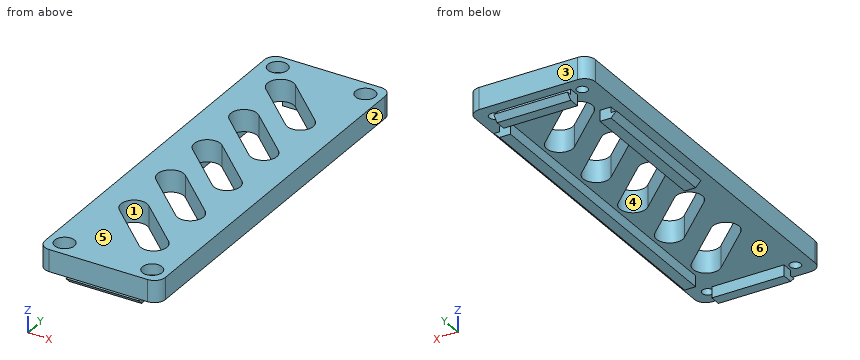
```python
from build123d import *

# Parameters (mm, degrees)
SKETCH_1_W          = 11
SKETCH_1_H          = 35
EXTRUDE_1_DEPTH     = 2
FILLET_1_R          = 1
SKETCH_2_W          = 1
SKETCH_2_H          = 27.801195883
SKETCH_2_H_2        = 12.696804569
SKETCH_2_W_2        = 6.728012357
SKETCH_2_H_3        = 1
SKETCH_2_W_3        = 6.596948746
EXTRUDE_2_DEPTH     = 1
SKETCH_3_W          = 6.641337803
SKETCH_3_H          = 0.5
EXTRUDE_3_DEPTH     = 0.5
SKETCH_4_W          = 0.5
SKETCH_4_H          = 12.696804569
EXTRUDE_4_DEPTH     = 0.5
SKETCH_5_W          = 6.728012357
SKETCH_5_H          = 0.5
EXTRUDE_5_DEPTH     = 0.5
SKETCH_6_W          = 0.5
SKETCH_6_H          = 27.801195883
EXTRUDE_6_DEPTH     = 0.5
CHAMFER_1_SIZE      = 0.5
CUT_EXTRUDE_1_REACH = 60.195
SKETCH_8_R          = 0.9
CUT_EXTRUDE_2_DEPTH = 1
SKETCH_9_R          = 0.5
CUT_EXTRUDE_3_DEPTH = 1


with BuildPart() as part:
    # 草图1 → 凸台-拉伸1 (new body)
    with BuildSketch(Plane.XY):
        with Locations((48.44429715, 4.125412508)):
            Rectangle(SKETCH_1_W, SKETCH_1_H)
    extrude(amount=EXTRUDE_1_DEPTH)

    # 圆角1
    fillet_1_edges = [part.edges().sort_by_distance(p)[0] for p in [
        (42.94429715, 21.625412508, 1),
        (53.94429715, 21.625412508, 1),
        (53.94429715, -13.374587492, 1),
        (42.94429715, -13.374587492, 1),
    ]]
    fillet(fillet_1_edges, radius=FILLET_1_R)

    # 草图2 → 凸台-拉伸2 (add)
    with BuildSketch(Plane(origin=(0, 0, 0), x_dir=(-1, 0, 0), z_dir=(0, 0, -1))):
        with Locations((-52.444918102, 4.669937054)):
            Rectangle(SKETCH_2_W, SKETCH_2_H)
        with Locations((-44.44429715, 10.285527485)):
            Rectangle(SKETCH_2_W, SKETCH_2_H_2)
        with Locations((-48.555014421, 20.125412508)):
            Rectangle(SKETCH_2_W_2, SKETCH_2_H_3)
        with Locations((-48.47250239, -11.874587492)):
            Rectangle(SKETCH_2_W_3, SKETCH_2_H_3)
    extrude(amount=EXTRUDE_2_DEPTH)

    # 草图3 → 凸台-拉伸3 (add)
    with BuildSketch(Plane.XZ.offset(12.374587492)):
        with Locations((48.494696919, -0.75)):
            Rectangle(SKETCH_3_W, SKETCH_3_H)
    extrude(amount=EXTRUDE_3_DEPTH)

    # 草图4 → 凸台-拉伸4 (add)
    with BuildSketch(Plane.ZY.offset(-43.94429715)):
        with Locations((-0.75, 10.285527485)):
            Rectangle(SKETCH_4_W, SKETCH_4_H)
    extrude(amount=EXTRUDE_4_DEPTH)

    # 草图5 → 凸台-拉伸5 (add)
    with BuildSketch(Plane(origin=(0, 20.625412508, 0), x_dir=(1, 0, 0), z_dir=(0, 1, 0))):
        with Locations((48.555014421, 0.75)):
            Rectangle(SKETCH_5_W, SKETCH_5_H)
    extrude(amount=EXTRUDE_5_DEPTH)

    # 草图6 → 凸台-拉伸6 (add)
    with BuildSketch(Plane(origin=(52.944918102, 0, 0), x_dir=(0, 0, -1), z_dir=(1, 0, 0))):
        with Locations((0.75, 4.669937054)):
            Rectangle(SKETCH_6_W, SKETCH_6_H)
    extrude(amount=EXTRUDE_6_DEPTH)

    # 倒角1
    chamfer_1_edges = [part.edges().sort_by_distance(p)[0] for p in [
        (48.494696919, -12.874587492, -1),
        (53.444918102, 4.669937054, -1),
        (48.555014421, 21.125412508, -1),
        (43.44429715, 10.285527485, -1),
    ]]
    chamfer(chamfer_1_edges, length=CHAMFER_1_SIZE - 0.0001)  # a hair under: the kernel refuses the full size

    # 草图7 → 切除-拉伸1 (cut, up to next)
    with BuildSketch(Plane.XY.offset(2), mode=Mode.PRIVATE) as cut_extrude_1_sk1:
        with BuildLine():
            Line((47.04721821, 18.494490282), (51.235350906, 14.562121415))
            ThreePointArc((51.235350906, 14.562121415), (51.288650219, 12.86986824), (49.596397044, 12.816568927))
            Line((49.596397044, 12.816568927), (45.408264348, 16.748937794))
            ThreePointArc((45.408264348, 16.748937794), (45.354965035, 18.441190969), (47.04721821, 18.494490282))
        make_face()
    cut_extrude_1_tool1 = extrude(cut_extrude_1_sk1.sketch, amount=-CUT_EXTRUDE_1_REACH, mode=Mode.PRIVATE) & part.part
    # 草图7 → 切除-拉伸1 (cut, up to next)
    with BuildSketch(Plane.XY.offset(2), mode=Mode.PRIVATE) as cut_extrude_1_sk2:
        with BuildLine():
            Line((45.408264348, 11.248937794), (49.596397044, 7.316568927))
            ThreePointArc((49.596397044, 7.316568927), (51.288650219, 7.36986824), (51.235350906, 9.062121415))
            Line((51.235350906, 9.062121415), (47.04721821, 12.994490282))
            ThreePointArc((47.04721821, 12.994490282), (45.354965035, 12.941190969), (45.408264348, 11.248937794))
        make_face()
    cut_extrude_1_tool2 = extrude(cut_extrude_1_sk2.sketch, amount=-CUT_EXTRUDE_1_REACH, mode=Mode.PRIVATE) & part.part
    # 草图7 → 切除-拉伸1 (cut, up to next)
    with BuildSketch(Plane.XY.offset(2), mode=Mode.PRIVATE) as cut_extrude_1_sk3:
        with BuildLine():
            Line((45.408264348, 5.748937794), (49.596397044, 1.816568927))
            ThreePointArc((49.596397044, 1.816568927), (51.288650219, 1.86986824), (51.235350906, 3.562121415))
            Line((51.235350906, 3.562121415), (47.04721821, 7.494490282))
            ThreePointArc((47.04721821, 7.494490282), (45.354965035, 7.441190969), (45.408264348, 5.748937794))
        make_face()
    cut_extrude_1_tool3 = extrude(cut_extrude_1_sk3.sketch, amount=-CUT_EXTRUDE_1_REACH, mode=Mode.PRIVATE) & part.part
    # 草图7 → 切除-拉伸1 (cut, up to next)
    with BuildSketch(Plane.XY.offset(2), mode=Mode.PRIVATE) as cut_extrude_1_sk4:
        with BuildLine():
            Line((45.408264348, 0.248937794), (49.596397044, -3.683431073))
            ThreePointArc((49.596397044, -3.683431073), (51.288650219, -3.63013176), (51.235350906, -1.937878585))
            Line((51.235350906, -1.937878585), (47.04721821, 1.994490282))
            ThreePointArc((47.04721821, 1.994490282), (45.354965035, 1.941190969), (45.408264348, 0.248937794))
        make_face()
    cut_extrude_1_tool4 = extrude(cut_extrude_1_sk4.sketch, amount=-CUT_EXTRUDE_1_REACH, mode=Mode.PRIVATE) & part.part
    # 草图7 → 切除-拉伸1 (cut, up to next)
    with BuildSketch(Plane.XY.offset(2), mode=Mode.PRIVATE) as cut_extrude_1_sk5:
        with BuildLine():
            Line((45.408264348, -5.251062206), (49.596397044, -9.183431073))
            ThreePointArc((49.596397044, -9.183431073), (51.288650219, -9.13013176), (51.235350906, -7.437878585))
            Line((51.235350906, -7.437878585), (47.04721821, -3.505509718))
            ThreePointArc((47.04721821, -3.505509718), (45.354965035, -3.558809031), (45.408264348, -5.251062206))
        make_face()
    cut_extrude_1_tool5 = extrude(cut_extrude_1_sk5.sketch, amount=-CUT_EXTRUDE_1_REACH, mode=Mode.PRIVATE) & part.part
    add(cut_extrude_1_tool1.solids().sort_by_distance((48.321808, 15.65553, 2))[0], mode=Mode.SUBTRACT)
    add(cut_extrude_1_tool2.solids().sort_by_distance((48.321808, 10.15553, 2))[0], mode=Mode.SUBTRACT)
    add(cut_extrude_1_tool3.solids().sort_by_distance((48.321808, 4.65553, 2))[0], mode=Mode.SUBTRACT)
    add(cut_extrude_1_tool4.solids().sort_by_distance((48.321808, -0.84447, 2))[0], mode=Mode.SUBTRACT)
    add(cut_extrude_1_tool5.solids().sort_by_distance((48.321808, -6.34447, 2))[0], mode=Mode.SUBTRACT)

    # 草图8 → 切除-拉伸2 (cut)
    with BuildSketch(Plane.XY.offset(2)):
        with Locations((44.44429715, 20.125412508)):
            Circle(SKETCH_8_R)
        with Locations((52.44429715, 20.125412508)):
            Circle(SKETCH_8_R)
        with Locations((44.44429715, -11.874587492)):
            Circle(SKETCH_8_R)
        with Locations((52.44429715, -11.874587492)):
            Circle(SKETCH_8_R)
    extrude(amount=-CUT_EXTRUDE_2_DEPTH, mode=Mode.SUBTRACT)

    # 草图9 → 切除-拉伸3 (cut)
    with BuildSketch(Plane.XY.offset(1)):
        with Locations((44.44429715, 20.125412508)):
            Circle(SKETCH_9_R)
        with Locations((52.44429715, 20.125412508)):
            Circle(SKETCH_9_R)
        with Locations((52.44429715, -11.874587492)):
            Circle(SKETCH_9_R)
        with Locations((44.44429715, -11.874587492)):
            Circle(SKETCH_9_R)
    extrude(amount=-CUT_EXTRUDE_3_DEPTH, mode=Mode.SUBTRACT)


solid = part.part
```
Work out the finished part from the listing and answer in its coordinate system (mm). Face numbers are marked on the shaded views. A direction names the side the tool comes from. Coordinates: 2 decimals unless noted, no trailing zeros. Loops run counter-clockwise (first coordinate to the right, second up) from the corner with the lowest first, then second, coordinate; pieces in that order, holes last. Notation, with made-up numbers: M -19.75,-16 L 2.25,-16 A33 cw 2.25,14 Z; hole C 82.25,-16.75 d11. An arc over 180 degrees is marked long. Use CSV: the item, a comma, the result in double quotes. Start each with the question number.
(1) Find section C-C, the plane z = 1.4. State how many separate pieces and enclosed holes the cut face has, then the cut area to 3 significant figures.
(2) Find section A-A, the plane x = 44.25. Give the vertices of the cut face in (y, z).
(3) Given pin 1 Ø2 at (x, y) = (44.5, 20.5) entering from +Z; pin 2 Ø0.8 at (y, z) = (-12, -0.5) entering from -X; pin 3 Ø1.4 at (x, y) = (52.44, -11.87) entering from +Z, each flat-ended and moving along its own axis, determine where each tip first touches the part or whether it passes through.
(4) For a pull along Y with two mould halves and no side action, classify the marked faces 1, 2, 3 and 4 as +Y half, -Y half, draft (parallel to the pull), parting line (faces both ways), or undercut.
(5) Consider line 1 (Y direction, x = 44.5, z = 0.65); line 2 (Y direction, x = 46.25, z = 1.5); line 3 (Y direction, x = 50.5, z = 0.75). Determine where each line is inside the solid, lowest interval first.
(6) For the marked faces 5 and 6, determine the directions among +Z, -Z, +X, -X, +Y, -Y from which every point of the face is accessible in a straight line to the end or side of a thin tool.
Recorded:
1,separate pieces,"1"
1,enclosed holes,"9"
1,area,"283 mm^2"
2,outline,"M -13.37,0 L -12.34,0 L -12.34,1 L -12.75,1 L -12.75,2 L -13.37,2 Z; M -11.41,0 L 3.94,0 L 3.94,-1 L 16.63,-1 L 16.63,0 L 19.66,0 L 19.66,1 L 19.25,1 L 19.25,2 L -11,2 L -11,1 L -11.41,1 Z; M 20.59,0 L 21.63,0 L 21.63,2 L 21,2 L 21,1 L 20.59,1 Z"
3,pin 1,"stops at z = 2"
3,pin 2,"stops at x = 45.17"
3,pin 3,"stops at z = 1"
4,face 1,"undercut"
4,face 2,"draft"
4,face 3,"+Y half"
4,face 4,"undercut"
5,line 1,"y = -13.37 to -12.37, -11.38 to 19.63, 20.62 to 21.63"
5,line 2,"y = -13.37 to -6.04, -3.18 to -0.54, 2.32 to 4.96, 7.82 to 10.46, 13.32 to 15.96, 18.82 to 21.63"
5,line 3,"y = -13.37 to -9.5, -6.75 to -4, -1.25 to 1.5, 4.25 to 7, 9.75 to 12.5, 15.25 to 21.63"
6,face 5,"+Z, +X, -X, +Y, -Y"
6,face 6,"none"
